Answer from the drawing. Dimensions are ordinates in mm from the lowest x, y and z of the part. A direction names the side the tool comes from. Give positions to 0.01 mm unless a question says otherwise; leave off trailing zeros. Loops run counter-clockwise (first coordinate to the right, second up) from the corner with the lowest first, then second, coordinate; pieces in that order, holes last. Notation, with made-up numbers: (58, 87) - (116, 87) arc R22 cw to (116, 125) - close; hole circle Ø2 at (-33, 71). An arc over 180 degrees is marked (long way). Write each question's results on one line, items separated by ' | '. Start each with the question number.
Q1. Find the intervals of material crossed by line 1 (Y direction, x = 2, z = 0.7); line 2 (X direction, y = 27, z = 0.9); line 3 (Z direction, x = 10, y = 33.5), in increasing order. Write a range as from..to.
Q2. The part is cut by section C-C, the plane y = 2. Write down the section's boundary in (x, z), plus the area to 3 significant figures.
Q3. The part is cut by section D-D, the plane x = 19.25. Write down the section's boundary in (y, z).
Q4. The part is cut by section A-A, the plane x = 2. Write down the section's boundary in (y, z), plus the area to 3 significant figures.
Q5. For the marked faces 1, 2 and 3, determine the directions among +Z, -Z, +X, -X, +Y, -Y from which every point of the face is accessible in a straight line to the end or side of a thin tool.
Q6. The part is cut by section B-B, the plane z = 1.45. Write down the section's boundary in (x, y), plus the area to 3 significant figures.
Q7. Given pin 1 (2.5 mm diameter, centred on y = 10, z = 1.5, fed in from +X); pin 2 (1 mm diameter, centred on x = 5.5, y = 25, fed in from -Z); pin 3 (3 mm diameter, centred on x = 17, z = 3.5, fed in from -Y), each flat-ended and moving along its own axis, determine where each tip first touches the part or whether it passes through.
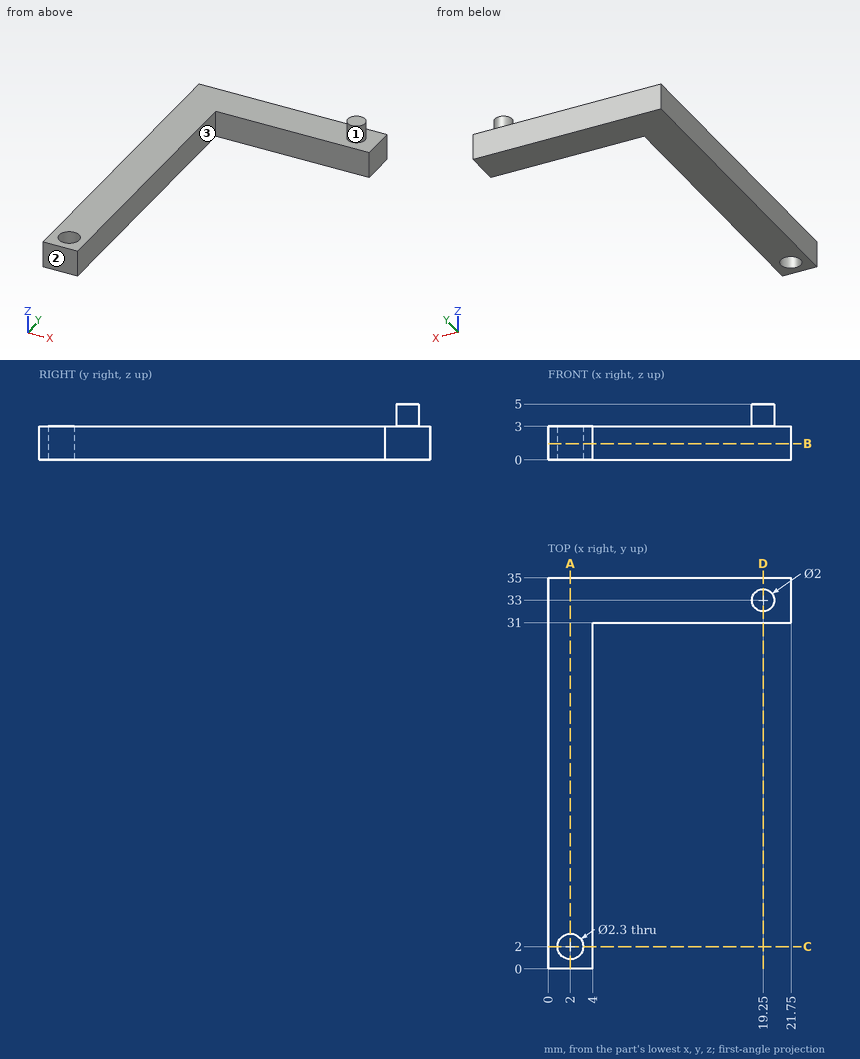
Check sheet entries:
1) line 1: y = 0..0.85, 3.15..35 | line 2: x = 0..4 | line 3: z = 0..3
2) outline: (0, 0) - (0.85, 0) - (0.85, 3) - (0, 3) - close; (3.15, 0) - (4, 0) - (4, 3) - (3.15, 3) - close | area: 5.10 mm^2
3) outline: (31, 0) - (35, 0) - (35, 3) - (34, 3) - (34, 5) - (32, 5) - (32, 3) - (31, 3) - close
4) outline: (0, 0) - (0.85, 0) - (0.85, 3) - (0, 3) - close; (3.15, 0) - (35, 0) - (35, 3) - (3.15, 3) - close | area: 98.1 mm^2
5) face 1: +Z | face 2: +Z, -Z, +X, -X, -Y | face 3: +Z, -Z, +X, -Y
6) outline: (0, 0) - (4, 0) - (4, 31) - (21.75, 31) - (21.75, 35) - (0, 35) - close; hole circle Ø2.3 at (2, 2) | area: 207 mm^2
7) pin 1: stops at x = 4 | pin 2: passes through | pin 3: stops at y = 31
